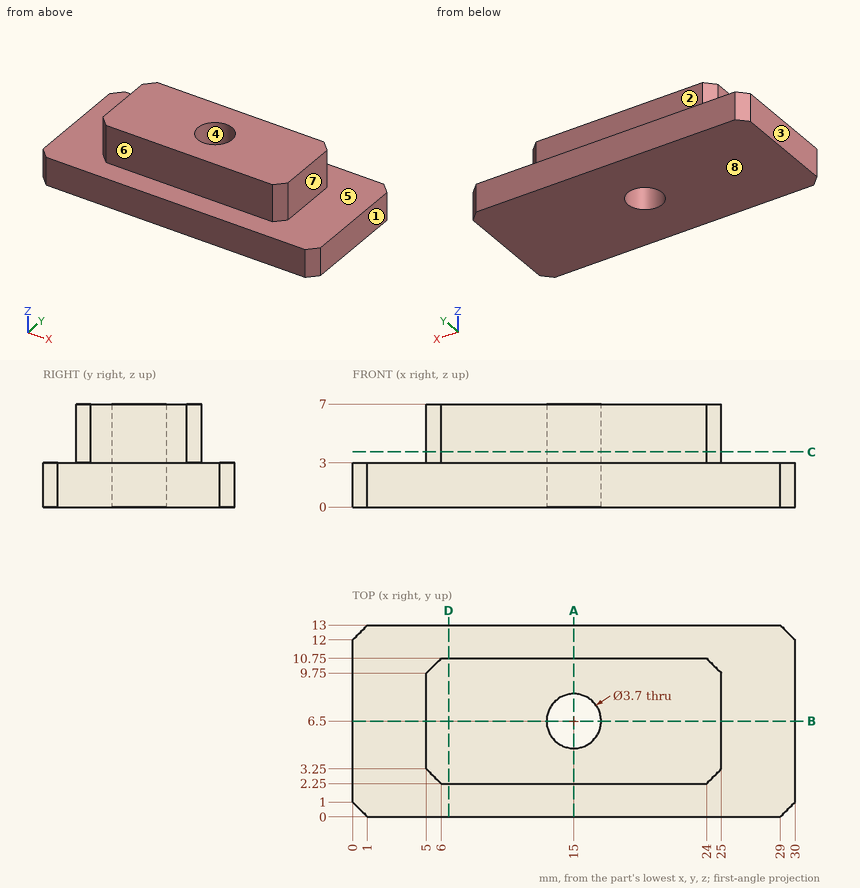
Source: three-view drawing plus pictorial views. Frame: mm from the lowest corner of the part. A direction names the side the tool comes from. Give positions to 0.01 mm unless a question says otherwise; leave off trailing zeros. Loops run counter-clockwise (first coordinate to the right, second up) from the corner with the lowest first, then second, coordinate; pieces in that order, holes last. Notation, with made-up numbers: (75, 2.25) -> (107, 2.25) arc R21 cw to (107, 17.25) -> close; hole circle Ø3 at (64, -30). An arc over 180 degrees is marked (long way). Put each result on its own line as item: value. Start each with the question number.
1) Cut plane B-B (y = 6.5). Return loops of the section in (x, z), then the cut area to 3 significant figures.
2) Cut plane C-C (z = 3.75). Return loops of the section in (x, y), then the cut area to 3 significant figures.
3) Draft query along X for the marked faces 1, 2, 3 and 4. Return one class per face: released by +X, released by -X, zero draft, split by the parting line, or undercut.
4) Cut plane A-A (x = 15). Return loops of the section in (y, z).
5) Reachability of the marked faces 5, 6, 7 and 8 from +Z, -Z, +X, -X, +Y, -Y: full face, straight path, thin tool, end or side. Return the list, or none.
6) Cut plane D-D (x = 6.5). Return loops of the section in (y, z).
7) Contact query for flat-ended pins moving along their axis: P1, Ø3, axis at x = 15, y = 6.5, coming from the +Z side; P2, Ø3, axis at x = 15, z = 5.5, coming from the +Y side; P3, Ø2, axis at y = 2.5, z = 5.5, coming from the -X side; P4, Ø3, axis at x = 12.5, z = 5, coming from the -Y side. Output: stop coordinate, or through.
8) Material intervals for probe 1 along Y at (x, z) = (15, 4); probe 2 along Y at (x, z) = (6.5, 6.25); probe 3 along Z at (x, y) = (1.75, 10.25), sorted ascending.
Results are:
1. outline: (0, 0) -> (13.15, 0) -> (13.15, 7) -> (5, 7) -> (5, 3) -> (0, 3) -> close; (16.85, 0) -> (30, 0) -> (30, 3) -> (25, 3) -> (25, 7) -> (16.85, 7) -> close
1. area: 144 mm2
2. outline: (5, 3.25) -> (6, 2.25) -> (24, 2.25) -> (25, 3.25) -> (25, 9.75) -> (24, 10.75) -> (6, 10.75) -> (5, 9.75) -> close; hole circle Ø3.7 at (15, 6.5)
2. area: 157 mm2
3. face 1: released by +X
3. face 2: zero draft
3. face 3: released by -X
3. face 4: undercut
4. outline: (0, 0) -> (4.65, 0) -> (4.65, 7) -> (2.25, 7) -> (2.25, 3) -> (0, 3) -> close; (8.35, 0) -> (13, 0) -> (13, 3) -> (10.75, 3) -> (10.75, 7) -> (8.35, 7) -> close
5. face 5: +Z
5. face 6: +Z, +X, -X, -Y
5. face 7: +Z, +X, +Y, -Y
5. face 8: -Z, +X, -X, +Y, -Y
6. outline: (0, 0) -> (13, 0) -> (13, 3) -> (10.75, 3) -> (10.75, 7) -> (2.25, 7) -> (2.25, 3) -> (0, 3) -> close
7. P1: passes through
7. P2: stops at y = 10.75
7. P3: stops at x = 5
7. P4: stops at y = 2.25
8. probe 1: y = 2.25 to 4.65, 8.35 to 10.75
8. probe 2: y = 2.25 to 10.75
8. probe 3: z = 0 to 3
